Work out the finished part from the listing and answer in its coordinate system (mm). A direction names the side the tool comes from. Coordinates: 2 decimals unless noted, no trailing zeros. Write each loop counter-clockwise with the first axis right and the second up, starting at its lowest first coordinate (ties: lowest second). Pieces come first, ordered by that corner, then holes. Notation, with made-up numbers: (-1, -22.5) - (15, -22.5) arc R11 ccw to (15, -10.5) - close; hole circle Ø6 at (5, 74.5). An arc over 180 degrees is marked (long way). One line per item, written item: value.
```python
from build123d import *

# Parameters (mm, degrees)
F1_DEPTH = 76.2
F2_DEPTH = 50.8
F3_DEPTH = 12.7
F4_DEPTH = 50.8
F5_DEPTH = 12.7


with BuildPart() as f1:
    # F0 (on Top) → F1 (new body)
    with BuildSketch(Plane.XY):
        with BuildLine():
            ThreePointArc((-190.5, 0), (0, -190.5), (190.5, 0))
            ThreePointArc((190.5, 0), (60.4014109978, 180.6707490146), (-152.1973181048, 114.5697445302))
            Line((-152.1973181048, 114.5697445302), (-132.2621264517, 99.5631081236))
            ThreePointArc((-132.2621264517, 99.5631081236), (52.4898806282, 157.0060349935), (165.5478256962, 0))
            ThreePointArc((165.5478256962, 0), (0, -165.5478256962), (-165.5478256962, 0))
            Line((-165.5478256962, 0), (-190.5, 0))
        make_face()
    extrude(amount=F1_DEPTH)

    # F0 (on Top) → F2 (join)
    with BuildSketch(Plane.XY):
        with BuildLine():
            ThreePointArc((165.5478256962, 0), (52.4898806282, 157.0060349935), (-132.2621264517, 99.5631081236))
            Line((-132.2621264517, 99.5631081236), (-98.495770837, 74.1447710289))
            ThreePointArc((-98.495770837, 74.1447710289), (39.0892796926, 116.9225904469), (123.2836726566, 0))
            ThreePointArc((123.2836726566, 0), (0, -123.2836726566), (-123.2836726566, 0))
            Line((-123.2836726566, 0), (-165.5478256962, 0))
            ThreePointArc((-165.5478256962, 0), (0, -165.5478256962), (165.5478256962, 0))
        make_face()
    extrude(amount=F2_DEPTH)

    # F0 (on Top) → F3 (join)
    with BuildSketch(Plane.XY):
        with BuildLine():
            ThreePointArc((123.2836726566, 0), (39.0892796926, 116.9225904469), (-98.495770837, 74.1447710289))
            Line((-98.495770837, 74.1447710289), (0, 0))
            Line((0, 0), (-123.2836726566, 0))
            ThreePointArc((-123.2836726566, 0), (0, -123.2836726566), (123.2836726566, 0))
        make_face()
    extrude(amount=F3_DEPTH)

    # F0 (on Top) → F4 (join)
    with BuildSketch(Plane.XY):
        with BuildLine():
            Line((-98.495770837, 74.1447710289), (-132.2621264517, 99.5631081236))
            ThreePointArc((-132.2621264517, 99.5631081236), (-157.0060349935, 52.4898806282), (-165.5478256962, 0))
            Line((-165.5478256962, 0), (-123.2836726566, 0))
            ThreePointArc((-123.2836726566, 0), (-116.9225904469, 39.0892796926), (-98.495770837, 74.1447710289))
        make_face()
    extrude(amount=F4_DEPTH)

    # F0 (on Top) → F5 (join)
    with BuildSketch(Plane.XY):
        with BuildLine():
            Line((0, 0), (-98.495770837, 74.1447710289))
            ThreePointArc((-98.495770837, 74.1447710289), (-116.9225904469, 39.0892796926), (-123.2836726566, 0))
            Line((-123.2836726566, 0), (0, 0))
        make_face()
    extrude(amount=F5_DEPTH)


solid = f1.part
```
Item 1: Section D-D, the plane y = 50 is taken. Determine the outline of the cut face in (x, z).
Evaluation:
outline: (-157.82, 0) - (183.82, 0) - (183.82, 76.2) - (157.82, 76.2) - (157.82, 50.8) - (112.69, 50.8) - (112.69, 12.7) - (-112.69, 12.7) - (-112.69, 50.8) - (-157.82, 50.8) - close
Item 2: Section A-A, the plane x = 0 is taken. Determine the outline of the cut face in (y, z), then the cut area to 3 significant figures.
Evaluation:
outline: (-190.5, 0) - (190.5, 0) - (190.5, 76.2) - (165.55, 76.2) - (165.55, 50.8) - (123.28, 50.8) - (123.28, 12.7) - (-123.28, 12.7) - (-123.28, 50.8) - (-165.55, 50.8) - (-165.55, 76.2) - (-190.5, 76.2) - close
area: 11,200 mm2
Item 3: Consider probe 1 along Y at (x, z) = (0, 35); probe 2 along Y at (x, z) = (0, 57.5); probe 3 along Z at (x, y) = (-152.5, -60.5). Determine where each line is inside the solid, lowest interval first.
Evaluation:
probe 1: y = -190.5 to -123.28, 123.28 to 190.5
probe 2: y = -190.5 to -165.55, 165.55 to 190.5
probe 3: z = 0 to 50.8
Item 4: Section C-C, the plane y = -18 is taken. Determine the outline of the cut face in (x, z), then the cut area to 3 significant figures.
Evaluation:
outline: (-189.65, 0) - (189.65, 0) - (189.65, 76.2) - (164.57, 76.2) - (164.57, 50.8) - (121.96, 50.8) - (121.96, 12.7) - (-121.96, 12.7) - (-121.96, 50.8) - (-164.57, 50.8) - (-164.57, 76.2) - (-189.65, 76.2) - close
area: 11,200 mm2
Item 5: Section B-B, the plane z = 33 is taken. Determine the outline of the cut face in (x, y), then the cut area to 3 significant figures.
Evaluation:
outline: (-190.5, 0) arc R190.5 ccw (long way) to (-152.2, 114.57) - (-132.26, 99.56) arc R165.55 ccw to (-165.55, 0) - close; hole circle Ø246.57 at (0, 0)
area: 63,400 mm2
Item 6: Given pin 1 (8 mm diameter, centred on y = -120, z = 50, fed in from -X); pin 2 (2 mm diameter, centred on x = 124, y = -49, fed in from +Z); pin 3 (3 mm diameter, centred on x = 116.5, z = 14.5, fed in from -Y), each flat-ended and moving along its own axis, determine where each tip first touches the part or whether it passes through.
Evaluation:
pin 1: stops at x = -151.11
pin 2: stops at z = 50.8
pin 3: stops at y = -151.87
Item 7: Which of the six approach directions +Z, -Z, +X, -X, +Y, -Y give full straight-line access (tool end or side, diameter ignored) to faces 1 (the face through (-56.888, -109.374, 31.483)), 2 (the face through (-3, 3, 0)), 3 (the face through (-156.767, 53.199, 25.044))?
Evaluation:
face 1: +Z
face 2: -Z, +X, -X, +Y, -Y
face 3: +Z, -Z, -X
Item 8: Determine the mould class of faces 4 (the face through (-2, 2, 12.7)), 5 (the face through (-178, 0, 38)), 6 (the face through (-123, -11, 50.8)), 7 (the face through (178.15, -67.48, 37.57)) for opening direction Y: +Y half, -Y half, draft (parallel to the pull), parting line (faces both ways), or undercut.
Evaluation:
face 4: undercut
face 5: +Y half
face 6: undercut
face 7: parting line
